from build123d import *

# Parameters (mm, degrees)
CYLINDER011_R     = 2.3
CYLINDER011_DEPTH = 39
CYLINDER010_R     = 2.3
CYLINDER010_DEPTH = 35
CYLINDER001_R     = 2.8
CYLINDER001_DEPTH = 60
CYLINDER003_R     = 2.8
CYLINDER003_DEPTH = 60
CYLINDER002_R     = 2.8
CYLINDER002_DEPTH = 60
CYLINDER_R        = 2.8
CYLINDER_DEPTH    = 60
PAD002_DEPTH      = 24


with BuildPart() as obj1:
    # Cylinder011 → Cylinder011 (new body)
    with BuildSketch(Plane(origin=(41, -12, -3), x_dir=(0, 0, 1), z_dir=(-1, 0, 0))):
        Circle(CYLINDER011_R)
    extrude(amount=CYLINDER011_DEPTH)


with BuildPart() as obj2:
    # Cylinder010 → Cylinder010 (new body)
    with BuildSketch(Plane(origin=(41, -12, 36), x_dir=(0, 0, 1), z_dir=(-1, 0, 0))):
        Circle(CYLINDER010_R)
    extrude(amount=CYLINDER010_DEPTH)


with BuildPart() as o2:
    # Cylinder001 → Cylinder001 (new body)
    with BuildSketch(Plane(origin=(41, -4, 36), x_dir=(0, 0, 1), z_dir=(-1, 0, 0))):
        Circle(CYLINDER001_R)
    extrude(amount=CYLINDER001_DEPTH)


with BuildPart() as u002:
    # Cylinder003 → Cylinder003 (new body)
    with BuildSketch(Plane(origin=(41, -20, -3), x_dir=(0, 0, 1), z_dir=(-1, 0, 0))):
        Circle(CYLINDER003_R)
    extrude(amount=CYLINDER003_DEPTH)


with BuildPart() as u001:
    # Cylinder002 → Cylinder002 (new body)
    with BuildSketch(Plane(origin=(41, -4, -3), x_dir=(0, 0, 1), z_dir=(-1, 0, 0))):
        Circle(CYLINDER002_R)
    extrude(amount=CYLINDER002_DEPTH)


with BuildPart() as o1:
    # Cylinder → Cylinder (new body)
    with BuildSketch(Plane(origin=(41, -20, 36), x_dir=(0, 0, 1), z_dir=(-1, 0, 0))):
        Circle(CYLINDER_R)
    extrude(amount=CYLINDER_DEPTH)


with BuildPart() as cut014:
    # Sketch → Pad002 (new body)
    with BuildSketch(Plane.XZ):
        with BuildLine():
            ThreePointArc((3.856276, 11.885302), (0.303894, 5.460599), (5.893532, 0.701169))
            Line((5.893532, 0.701169), (5.893532, -8.298831))
            Line((5.893532, -8.298831), (1.893532, -8.298831))
            Line((1.893532, -8.298831), (-4.873896, -7.706757))
            Line((-4.873896, -7.706757), (-4.873896, 40.051511))
            Line((-4.873896, 40.051511), (5.893532, 40.993539))
            Line((5.893532, 40.993539), (9.893532, 40.993539))
            Line((9.893532, 40.993539), (9.893532, 31.993539))
            add(Edge.make_bspline(
                [(9.893532, 31.993539), (-25.2112, 31.993539), (3.856276, 11.885302)],
                knots=[0, 0, 0, 2.546366, 2.546366, 2.546366], degree=2, weights=[1, 0.293239, 1]))
        make_face()
    extrude(amount=PAD002_DEPTH)

    # Cut: cut O1
    add(o1.part, mode=Mode.SUBTRACT)

    # Cut010: cut U001
    add(u001.part, mode=Mode.SUBTRACT)

    # Cut011: cut U002
    add(u002.part, mode=Mode.SUBTRACT)

    # Cut012: cut O2
    add(o2.part, mode=Mode.SUBTRACT)

    # Cut013: cut obj2
    add(obj2.part, mode=Mode.SUBTRACT)

    # Cut014: cut obj1
    add(obj1.part, mode=Mode.SUBTRACT)


solid = cut014.part
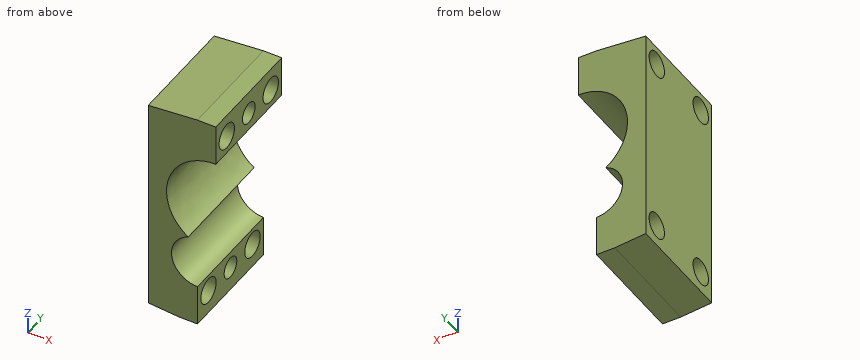
Model file for the job. Use its own axes, mm. Round coordinates to 2 decimals unless told otherwise and drop trailing zeros. Order: outer loops, then holes, each group sorted by start corner. A loop starts at its lowest first (then second) coordinate and runs counter-clockwise, first axis right, second up. Notation, with made-up numbers: M 50.25,84 L 92.25,84 A15 ccw 92.25,102 Z; hole C 59,-38.75 d5. An arc over 180 degrees is marked long. Write each question's results on one line, items separated by ' | '. Start each with the question number.
(1) Saw through at C-C, the plane z = -3. Give the cut face in (x, y).
(2) Saw through at D-D, the plane x = 4.5. State how many separate pieces and enclosed holes the cut face has, then the cut area to 3 significant figures.
(3) Drop flat-ended pins along their axis: pin 1 (1.5 mm diameter, centred on x = -2, z = 11, fed in from +Y); pin 2 (7 mm diameter, centred on y = -15, z = -4, fed in from +X); pin 3 (1.4 mm diameter, centred on y = -12, z = -2.5, fed in from +X); pin 4 (8 mm diameter, centred on y = -21.5, z = 20, fed in from +X). Give the stop position or say it passes through.
(4) Probe probe 1 along Y at (x, z) = (3.3, -3); probe 2 along Y at (x, z) = (3, 36); probe 3 along Z at (x, y) = (5, -19.5) (3 decimals). List the from-to ranges inside material, lowest first. Write a range as from..to.
(5) Saw through at B-B, the plane x = -1.5. Give the cut face in (y, z), then the cut area to 3 significant figures.
(6) Saw through at A-A, the plane z = 36. Give the cut face in (x, y).
Established:
1) outline: M -4.87,-24 L 5.89,-24 L 5.89,-22.8 L -4.87,-22.8 Z; M -4.87,-17.2 L 5.89,-17.2 L 5.89,-14.3 L 2,-14.3 L 2,-9.7 L 5.89,-9.7 L 5.89,-6.8 L -4.87,-6.8 Z; M -4.87,-1.2 L 5.89,-1.2 L 5.89,0 L -4.87,0 Z
2) separate pieces: 2 | enclosed holes: 5 | area: 354 mm^2
3) pin 1: stops at y = 0 | pin 2: stops at x = 5.89 | pin 3: stops at x = 2 | pin 4: stops at x = 0.3
4) probe 1: y = -24..-22.8, -17.2..-14.3, -9.7..-6.8, -1.2..0 | probe 2: y = -24..-22.8, -17.2..-6.8, -1.2..0 | probe 3: z = -8.299..-5.755, -0.245..0.789, 30.792..33.245, 38.755..40.915
5) outline: M -24,-8 L 0,-8 L 0,40.35 L -24,40.35 Z; hole C -20,-3 d5.6; hole C -20,36 d5.6; hole C -4,-3 d5.6; hole C -4,36 d5.6 | area: 1,060 mm^2
6) outline: M -4.87,-24 L 9.89,-24 L 9.89,-22.8 L -4.87,-22.8 Z; M -4.87,-17.2 L 9.89,-17.2 L 9.89,-14.3 L 6,-14.3 L 6,-9.7 L 9.89,-9.7 L 9.89,-6.8 L -4.87,-6.8 Z; M -4.87,-1.2 L 9.89,-1.2 L 9.89,0 L -4.87,0 Z
